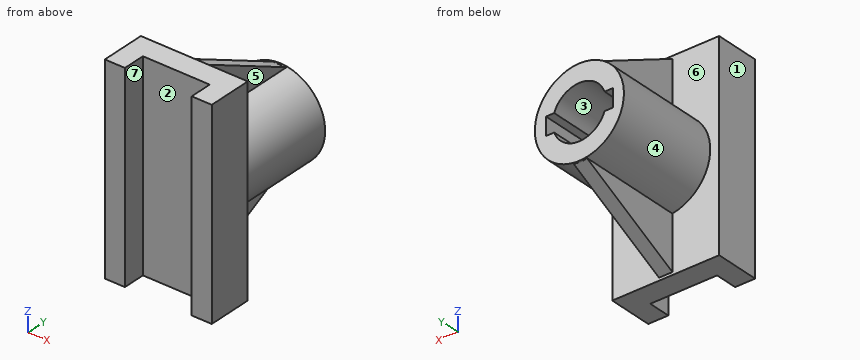
from build123d import *

# Parameters (mm, degrees)
EXTRUDE_1_DEPTH = 90
SKETCH_2_R      = 20
EXTRUDE_2_DEPTH = 48
RIB_44_REACH    = 117.326
SKETCH_5_WALL_W = 285.43665717
SKETCH_5_WALL_H = 6
RIB_45_REACH    = 117.326
SKETCH_7_WALL_W = 285.43665717
SKETCH_7_WALL_H = 6


with BuildPart() as part:
    # Эскиз1 → Бобышка-Вытянуть1 (new body)
    with BuildSketch(Plane.XY):
        Polygon((-15, 0), (-15, 10), (15, 10), (15, 0), (24, 0), (24, 20), (-24, 20), (-24, 0), align=None)
    extrude(amount=-EXTRUDE_1_DEPTH)

    # Эскиз2 → Бобышка-Вытянуть2 (add)
    with BuildSketch(Plane(origin=(0, 20, 0), x_dir=(1, 0, 0), z_dir=(0, 1, 0))):
        with Locations(Location((0, 45, 0), (0, 0, 270))):
            Circle(SKETCH_2_R)
        with BuildLine():
            Line((-11.313708499, 49), (-15, 49))
            Line((-15, 49), (-15, 41))
            Line((-15, 41), (-11.313708499, 41))
            ThreePointArc((-11.313708499, 41), (0, 33), (11.313708499, 41))
            Line((11.313708499, 41), (15, 41))
            Line((15, 41), (15, 49))
            Line((15, 49), (11.313708499, 49))
            ThreePointArc((11.313708499, 49), (0, 57), (-11.313708499, 49))
        make_face(mode=Mode.SUBTRACT)
    extrude(amount=EXTRUDE_2_DEPTH)

    # Эскиз5 wall → Ребро44 (add, up to next)
    with BuildSketch(Plane(origin=(0, 43.563200657, -13.108782301), x_dir=(0, -0.892792260785, 0.45046862164), z_dir=(0, -0.45046862164, -0.892792260785)), mode=Mode.PRIVATE) as rib_44_sk1:
        Rectangle(SKETCH_5_WALL_W, SKETCH_5_WALL_H)
    rib_44_tool1 = extrude(rib_44_sk1.sketch, amount=RIB_44_REACH, mode=Mode.PRIVATE) - part.part
    add(rib_44_tool1.solids().sort_by_distance((0, 43.563200657, -13.108782301))[0])

    # Эскиз7 wall → Ребро45 (add, up to next)
    with BuildSketch(Plane(origin=(0, 43.563200657, -76.889084379), x_dir=(0, -0.892792260785, -0.45046862164), z_dir=(0, 0.45046862164, -0.892792260785)), mode=Mode.PRIVATE) as rib_45_sk1:
        Rectangle(SKETCH_7_WALL_W, SKETCH_7_WALL_H)
    rib_45_tool1 = extrude(rib_45_sk1.sketch, amount=-RIB_45_REACH, mode=Mode.PRIVATE) - part.part
    add(rib_45_tool1.solids().sort_by_distance((0, 43.563200657, -76.889084379))[0])


solid = part.part
The listing builds one solid part. Answer for the finished solid, in the listing's coordinates (mm). Face numbers are marked on the shaded views. A direction names the side the tool comes from. Round coordinates to 2 decimals unless told otherwise and drop trailing zeros. Write each loop counter-clockwise with the first axis right and the second up, starting at its lowest first coordinate (ties: lowest second). Pieces come first, ordered by that corner, then holes. Notation, with made-up numbers: M -33,-27 L 0,-27 A23 cw 0,-14 Z; hole C 47,35 d7. An arc over 180 degrees is marked long. Write each question's results on one line, items separated by ' | '. Start each with the question number.
Item 1: A cutting plane is placed at B-B on y = 35.5. Write down the section's boundary in (x, z), and give its area (3 significant figures).
Item 2: For a pull along X with two mould halves and no side action, classify the marked faces 1, 2, 3 and 4 as pulls with the +X half, pulls with the -X half, needs draft (parallel to the pull), parting line crosses it, or undercut.
Item 3: For the marked faces 5, 6 and 7, determine the directions among +Z, -Z, +X, -X, +Y, -Y from which every point of the face is accessible in a straight line to the end or side of a thin tool.
Item 4: Flat-ended cylindrical pins translate along their axes: pin 1 Ø3 at (x, y) = (13.5, 59) entering from -Z; pin 2 Ø1.5 at (x, z) = (-4, -15.5) entering from -Y; pin 3 Ø3 at (x, y) = (-7.5, 38) entering from -Z. Find the tip coordinate at first contact, or state that the pin passes through.
Item 5: A cutting plane is placed at D-D on z = -61. Write down the section's boundary in (x, y).
Item 6: A cutting plane is placed at C-C on x = -13. Write down the section's boundary in (y, z), and give its area (3 significant figures).
Item 7: Straight lines are drawn through the part: L1, parallel to X at y = 8.5, z = -70.5; L2, parallel to Y at x = 9.5, z = -46; L3, parallel to X at y = 56, z = -23. For each, find the intervals that lie inside material, in ascending order. Write a range as [from, to].
Item 8: A cutting plane is placed at A-A on z = -45. Write down the section's boundary in (x, y), and give its area (3 significant figures).
Check sheet entries:
1) outline: M -3,-80.96 L 3,-80.96 L 3,-64.77 A20 ccw 3,-25.23 L 3,-9.04 L -3,-9.04 L -3,-25.23 A20 ccw -3,-64.77 Z; hole M -15,-49 L -11.31,-49 A12 ccw 11.31,-49 L 15,-49 L 15,-41 L 11.31,-41 A12 ccw -11.31,-41 L -15,-41 Z | area: 945 mm²
2) face 1: pulls with the -X half | face 2: undercut | face 3: undercut | face 4: parting line crosses it
3) face 5: +Z, +X, +Y | face 6: +Y | face 7: +Z, -Z, -Y
4) pin 1: z = -61 | pin 2: y = 10 | pin 3: z = -64.08
5) outline: M -24,0 L -15,0 L -15,10 L 15,10 L 15,0 L 24,0 L 24,20 L 12,20 L 12,68 L -12,68 L -12,20 L -24,20 Z
6) outline: M 10,-90 L 20,-90 L 20,-60.2 L 68,-60.2 L 68,-49 L 20,-49 L 20,-41 L 68,-41 L 68,-29.8 L 20,-29.8 L 20,0 L 10,0 Z | area: 1,980 mm²
7) L1: [-24, -15], [15, 24] | L2: [10, 20] | L3: [-3, 3]
8) outline: M -24,0 L -15,0 L -15,10 L 15,10 L 15,0 L 24,0 L 24,20 L 20,20 L 20,68 L 15,68 L 15,20 L -15,20 L -15,68 L -20,68 L -20,20 L -24,20 Z | area: 1,140 mm²
